For this review, use the dimensioned drawing (mm, ordinates from the lowest corner) and the shaded views. Give positions to 0.01 mm unless a question says otherwise; leave off trailing zeros. Loops run counter-clockwise (first coordinate to the right, second up) from the corner with the lowest first, then second, coordinate; pieces in that order, holes last. Notation, with made-up numbers: (88, 30) -> (128, 30) arc R13 cw to (128, 35) -> close; hole circle Ø3 at (-7.75, 47). An arc over 180 degrees is marked (long way). Write each question's results on one line, items separated by ' | '. Start each with the question number.
Q1. We need section A-A (z = 7). Write out the cut boundary in (x, y), plus the area to 3 significant figures.
Q2. We need section D-D (x = 12.5). Write out the cut boundary in (y, z).
Q3. Mouldability with a two-part tool opening along Z and no side actions: class the marked faces 1 and 2 as released by +Z, released by -Z, zero draft, split by the parting line, or undercut.
Q4. Insertion check: pin 1 Ø0.8 at (y, z) = (6.5, 64) entering from +X; pin 2 Ø1 at (x, z) = (19, 15) entering from +Y; pin 3 Ø0.8 at (x, z) = (0.5, 53) entering from +Y. Each pin has a flat end and moves straight along its axis. Give the tip position at first contact, or say it passes through.
Q5. We need section B-B (x = 52). Write out the cut boundary in (y, z).
Q6. Wall thickness on L1, parallel to Z at x = 22.5, y = 4.5; L2, parallel to Z at x = 55.5, y = 3.25; L3, parallel to X at y = 2.5, z = 27: over which ranges is each line inside the solid? List them lowest first. Write a range as [from, to].
Q7. We need section C-C (y = 4.5). Write out the cut boundary in (x, z), plus the area to 3 significant figures.
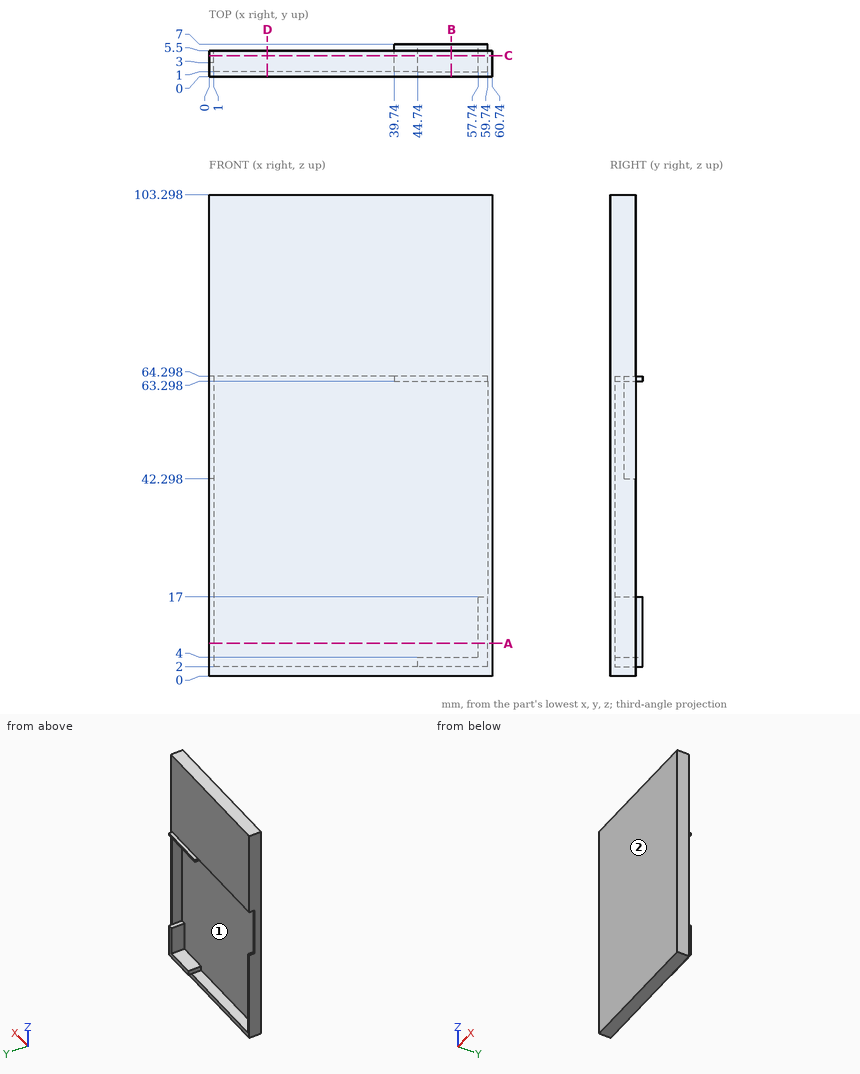
Output:
1) outline: (0, 0) -> (60.74, 0) -> (60.74, 5.5) -> (59.74, 5.5) -> (59.74, 7) -> (57.74, 7) -> (57.74, 1) -> (1, 1) -> (1, 5.5) -> (0, 5.5) -> close | area: 81.7 mm2
2) outline: (0, 0) -> (5.5, 0) -> (5.5, 2) -> (1, 2) -> (1, 64.3) -> (5.5, 64.3) -> (5.5, 103.3) -> (0, 103.3) -> close
3) face 1: undercut | face 2: zero draft
4) pin 1: x = 59.74 | pin 2: y = 1 | pin 3: y = 3
5) outline: (0, 0) -> (5.5, 0) -> (5.5, 2) -> (7, 2) -> (7, 4) -> (1, 4) -> (1, 63.3) -> (7, 63.3) -> (7, 64.3) -> (5.5, 64.3) -> (5.5, 103.3) -> (0, 103.3) -> close
6) L1: [0, 2], [64.3, 103.3] | L2: [0, 4], [63.3, 103.3] | L3: [0, 1], [59.74, 60.74]
7) outline: (0, 0) -> (60.74, 0) -> (60.74, 103.3) -> (0, 103.3) -> (0, 64.3) -> (39.74, 64.3) -> (39.74, 63.3) -> (59.74, 63.3) -> (59.74, 17) -> (57.74, 17) -> (57.74, 4) -> (44.74, 4) -> (44.74, 2) -> (1, 2) -> (1, 42.3) -> (0, 42.3) -> close | area: 2,670 mm2
